```python
from build123d import *

# Parameters (mm, degrees)
SKETCH_1_W                  = 20
SKETCH_1_H                  = 20
SKETCH_1_W_2                = 17
SKETCH_1_H_2                = 17
EXTRUDE_1_DEPTH             = 540
SKETCH_3_R                  = 2.25
CUT_EXTRUDE_2_DEPTH         = 20
HOLE_WIZARD_5_4_5_4_1_D     = 5.4
HOLE_WIZARD_10_0_10_1_D     = 10
HOLE_WIZARD_10_0_10_1_DEPTH = 1.5


with BuildPart() as part:
    # ｽｹｯﾁ1 → ﾎﾞｽ - 押し出し1 (new body)
    with BuildSketch(Plane.XY):
        Rectangle(SKETCH_1_W, SKETCH_1_H)
        Rectangle(SKETCH_1_W_2, SKETCH_1_H_2, mode=Mode.SUBTRACT)
    extrude(amount=EXTRUDE_1_DEPTH)

    # ｽｹｯﾁ3 → ｶｯﾄ - 押し出し2 (cut)
    with BuildSketch(Plane(origin=(10, 0, 0), x_dir=(0, 0, -1), z_dir=(1, 0, 0))):
        with Locations((-530, 0)):
            Circle(SKETCH_3_R)
        with Locations((-438, 0)):
            Circle(SKETCH_3_R)
        with Locations((-102, 0)):
            Circle(SKETCH_3_R)
        with Locations((-10, 0)):
            Circle(SKETCH_3_R)
    extrude(amount=-CUT_EXTRUDE_2_DEPTH, mode=Mode.SUBTRACT)

    # Ø5.4 (5.4) 直径の穴1 (through all)
    with Locations(Plane(origin=(0, 10, 0), x_dir=(1, 0, 0), z_dir=(0, 1, 0))):
        with Locations((0, -148), (0, -190), (0, -350), (0, -392)):
            Hole(HOLE_WIZARD_5_4_5_4_1_D / 2)

    # Ø10.0 (10) 直径の穴1
    with Locations(Plane(origin=(0, -10, 0), x_dir=(-1, 0, 0), z_dir=(0, -1, 0))):
        with Locations((0, -148), (0, -190), (0, -350), (0, -392)):
            Hole(HOLE_WIZARD_10_0_10_1_D / 2, depth=HOLE_WIZARD_10_0_10_1_DEPTH)


solid = part.part
```
Model file for the job. Use its own axes, mm. A direction names the side the tool comes from. Round coordinates to 2 decimals unless told otherwise and drop trailing zeros. Loops run counter-clockwise (first coordinate to the right, second up) from the corner with the lowest first, then second, coordinate; pieces in that order, holes last. Notation, with made-up numbers: M -30,45 L -4,45 A11 ccw -4,57 Z; hole C -38,22.25 d3. An arc over 180 degrees is marked long. Put each result on its own line as item: value. Start each with the question number.
Item 1: 3-axis set-ups, long thin cutter, end or side, ignore diameter. For faces 4 (the face through (-0.651, -9.24, 185.043)), 5 (the face through (0, -8.5, 266)), 6 (the face through (-10, 0, 266)): which of +Z, -Z, +X, -X, +Y, -Y reach the whole face in a straight line?
Item 2: Cut at A-A (y = 5.25). List the corners of the cut face in (x, z), then the cut area to 3 significant figures.
Item 3: Drill centre lines: line 1 along Z through (x, y) = (0, -8.75); line 2 along X through (y, z) = (9.55, 392); line 3 along X through (y, z) = (1, 345.5). Where is each one in solid material? Low to high.
Item 4: Drop flat-ended pins along their axis: P1, Ø7, axis at y = 0, z = 438, coming from the -X side; P2, Ø2, axis at x = 1.5, y = -6.5, coming from the +Z side; P3, Ø9, axis at x = 0, z = 392, coming from the -Y side. Give the stop position or say it passes through.
Item 5: Cut at B-B (z = 91.5). List the corners of the cut face in (x, y), then the cut area to 3 significant figures.
Item 6: Mould opens along Y. For faces 1 (the face through (-9, 0, 540)), 2 (the face through (0, 8.5, 266)), 3 (the face through (0, -10, 266)) say: released by +Y, released by -Y, zero draft, split by the parting line, or undercut.
Answer block:
1. face 4: -Y
1. face 5: +Z, -Z
1. face 6: +Z, -Z, -X, +Y, -Y
2. outline: M -10,0 L -8.5,0 L -8.5,540 L -10,540 Z; M 8.5,0 L 10,0 L 10,540 L 8.5,540 Z
2. area: 1,620 mm2
3. line 1: 0 to 143, 153 to 185, 195 to 345, 355 to 387, 397 to 540
3. line 2: -10 to -2.7, 2.7 to 10
3. line 3: -10 to -8.5, 8.5 to 10
4. P1: x = -10
4. P2: through
4. P3: y = 8.5
5. outline: M -10,-10 L 10,-10 L 10,10 L -10,10 Z; hole M -8.5,-8.5 L 8.5,-8.5 L 8.5,8.5 L -8.5,8.5 Z
5. area: 111 mm2
6. face 1: zero draft
6. face 2: undercut
6. face 3: released by -Y
